Build history of the part. All positions in model axes, mm. A direction names the side the tool comes from. Coordinates: 2 decimals unless noted, no trailing zeros. Order: outer loops, then holes, each group sorted by start corner. A loop starts at its lowest first (then second) coordinate and runs counter-clockwise, first axis right, second up. Notation, with made-up numbers: M 13.25,70.25 L 33.25,70.25 A24 ccw 33.25,93.25 Z; hole C 22,-26.5 d6. An arc over 180 degrees is marked long. Write item = value, one per line. Start each with the question number.
Q1. Band-saw the part on A-A on x = 82. Write the cut outline in (y, z).
Q2. 3-axis set-ups, long thin cutter, end or side, ignore diameter. For faces 1 (the face through (-0.021, -62.935, 6.204)), 2 (the face through (80.5, -4.4, 3)), 3 (the face through (33, 0, 20)): which of +Z, -Z, +X, -X, +Y, -Y reach the whole face in a straight line?
Q3. Band-saw the part on D-D on x = 0. State how many separate pieces and enclosed holes the cut face has, plus the area to 3 significant figures.
Q4. Band-saw the part on C-C on z = 55.5. Write the cut outline in (x, y), plus the area to 3 significant figures.
Q5. Drill centre lines: probe 1 along Y at (x, z) = (0, 0.55); probe 2 along Y at (x, z) = (25.3, 55.5); probe 3 along Z at (x, y) = (25.55, 0). Where is each one in solid material? Low to high.
Q6. Pull direction X, two halves, no side cores. Call faces 4 (the face through (15, 16, 7)), 5 (the face through (0, -33, 20)), 6 (the face through (-25, 0, 10)): released by +X, released by -X, zero draft, split by the parting line, or undercut.
Q7. Pin check, flat tips, straight feed: P1, Ø11, axis at y = -39.5, z = 14.5, coming from the +X side; P2, Ø4, axis at y = 22.5, z = 17.5, coming from the +X side; P3, Ø2.5, axis at x = -3.5, z = 17.5, coming from the -Y side; P4, Ø3.5, axis at x = 23, y = 19, coming from the -Z side. Stop position of each tip, or through.
```python
from build123d import *

# Parameters (mm, degrees)
CROQUIS2_W                                           = 50
CROQUIS2_H                                           = 50
CROQUIS2_R                                           = 3.5
SALIENTE_EXTRUIR2_DEPTH                              = 20
CROQUIS3_R                                           = 7.5
CORTAR_EXTRUIR1_DEPTH                                = 3
SALIENTE_EXTRUIR3_DEPTH                              = 40
SALIENTE_EXTRUIR4_DEPTH                              = 2.65
CORTAR_EXTRUIR2_START                                = -2
CORTAR_EXTRUIR2_DEPTH                                = 5
CORTAR_EXTRUIR5_START                                = -2.65
CORTAR_EXTRUIR5_DEPTH                                = 2.65
SALIENTE_EXTRUIR5_DEPTH                              = 44.75
CROQUIS13_R                                          = 3
CORTAR_EXTRUIR6_DEPTH                                = 15.2
SALIENTE_EXTRUIR6_START                              = -21.5
SALIENTE_EXTRUIR6_DEPTH                              = 13
SALIENTE_EXTRUIR7_START                              = -5
SALIENTE_EXTRUIR7_DEPTH                              = 3
REDONDEO1_R                                          = 2
CROQUIS17_R                                          = 2
CORTAR_EXTRUIR7_DEPTH                                = 3
CROQUIS18_R                                          = 2
CORTAR_EXTRUIR8_DEPTH                                = 3
REFRENTADO_PARA_TORNILLO_TAP_N_CON_CABEZ_D           = 4.5
REFRENTADO_PARA_TORNILLO_TAP_N_CON_CABEZ_CSINK_D     = 8.96
REFRENTADO_PARA_TORNILLO_TAP_N_CON_CABEZ_CSINK_ANGLE = 90
REDONDEO1_OF_SIMETR_A3_R                             = 2


with BuildPart() as part:
    # Croquis2 → Saliente-Extruir2 (new body)
    with BuildSketch(Plane.XY):
        Rectangle(CROQUIS2_W, CROQUIS2_H)
        Circle(CROQUIS2_R, mode=Mode.SUBTRACT)
    extrude(amount=SALIENTE_EXTRUIR2_DEPTH)

    # Croquis3 → Cortar-Extruir1 (cut)
    with BuildSketch(Plane.XY.offset(20)):
        Circle(CROQUIS3_R)
    extrude(amount=-CORTAR_EXTRUIR1_DEPTH, mode=Mode.SUBTRACT)

    # Croquis4 → Saliente-Extruir3 (add)
    with BuildSketch(Plane(origin=(0, 0, 0), x_dir=(-1, 0, 0), z_dir=(0, 0, -1))):
        Polygon((-25, -25), (-25, 17.4), (-28, 17.4), (-28, -28), (17.4, -28), (17.4, -25), align=None)
    extrude(amount=-SALIENTE_EXTRUIR3_DEPTH)

    # Croquis5 → Saliente-Extruir4 (add)
    with BuildSketch(Plane(origin=(0, 17.4, 0), x_dir=(1, 0, 0), z_dir=(0, 1, 0))):
        Polygon((25, 0), (51, 0), (25, -25), align=None)
    saliente_extruir4 = extrude(amount=-SALIENTE_EXTRUIR4_DEPTH)

    # Croquis6 → Cortar-Extruir2 (cut)
    with BuildSketch(Plane.XZ.offset(-14.75).offset(CORTAR_EXTRUIR2_START)):
        Polygon((44.824955825, 4.550258722), (30.300169567, 18.516399355), (26.037550962, 14.083276006), (40.56233722, 0.117135373), align=None)
    cortar_extruir2 = extrude(amount=CORTAR_EXTRUIR2_DEPTH, mode=Mode.SUBTRACT)

    # Simetría2: Saliente-Extruir4, Cortar-Extruir2 across plane
    add(saliente_extruir4.mirror(Plane(origin=(0, 0, 0), x_dir=(0, 0, 1), z_dir=(0.707106781, 0.707106781, 0))))
    add(cortar_extruir2.mirror(Plane(origin=(0, 0, 0), x_dir=(0, 0, 1), z_dir=(0.707106781, 0.707106781, 0))), mode=Mode.SUBTRACT)

    # Croquis11 → Cortar-Extruir5 (cut)
    with BuildSketch(Plane.XZ.offset(-14.75).offset(CORTAR_EXTRUIR5_START)):
        Polygon((28, 0), (51, 0), (28, 22.115384615), align=None)
    extrude(amount=CORTAR_EXTRUIR5_DEPTH, mode=Mode.SUBTRACT)

    # Croquis14 → Saliente-Extruir5 (add)
    with BuildSketch(Plane.XZ.offset(-16.75)):
        Polygon((26.037550962, 14.083276006), (28, 12.196305777), (28, 16.124223005), align=None)
    extrude(amount=SALIENTE_EXTRUIR5_DEPTH)

    # Croquis13 → Cortar-Extruir6 (cut)
    with BuildSketch(Plane(origin=(0, 0, 0), x_dir=(-1, 0, 0), z_dir=(0, 0, -1))):
        with BuildLine():
            Line((-25, 25), (-14, 25))
            Line((-14, 25), (-14, 19))
            ThreePointArc((-14, 19), (-15.464466094, 15.464466094), (-19, 14))
            Line((-19, 14), (-25, 14))
            Line((-25, 14), (-28, 14))
            Line((-28, 14), (-28, 17.4))
            Line((-28, 17.4), (-25, 17.4))
            Line((-25, 17.4), (-25, 25))
        make_face()
        with Locations((-19.802765158, 19.802765158)):
            Circle(CROQUIS13_R, mode=Mode.SUBTRACT)
    extrude(amount=-CORTAR_EXTRUIR6_DEPTH, mode=Mode.SUBTRACT)

    # Croquis15 → Saliente-Extruir6 (add)
    with BuildSketch(Plane.XZ.offset(28).offset(SALIENTE_EXTRUIR6_START)):
        Polygon((28, 0), (78, 0), (89, 0), (89, 3), (75, 3), (28, 50), (28, 61), (25, 61), (25, 40), (28, 40), align=None)
        Polygon((31, 42.757359313), (70.757359313, 3), (31, 3), align=None, mode=Mode.SUBTRACT)
    saliente_extruir6 = extrude(amount=-SALIENTE_EXTRUIR6_DEPTH)

    # Croquis16 → Saliente-Extruir7 (add)
    with BuildSketch(Plane.XZ.offset(6.5).offset(SALIENTE_EXTRUIR7_START)):
        Polygon((31, 3), (70.757359313, 3), (31, 42.757359313), align=None)
        Polygon((33, 5), (65.928932188, 5), (33, 37.928932188), align=None, mode=Mode.SUBTRACT)
    saliente_extruir7 = extrude(amount=-SALIENTE_EXTRUIR7_DEPTH)

    # Redondeo1
    redondeo1_edges = [part.edges().sort_by_distance(p)[0] for p in [
        (33, 0, 37.928932188),
        (65.928932188, 0, 5),
        (33, 0, 5),
    ]]
    fillet(redondeo1_edges, radius=REDONDEO1_R)

    # Croquis17 → Cortar-Extruir7 (cut)
    with BuildSketch(Plane.XY.offset(3)):
        with Locations((82, 0)):
            Circle(CROQUIS17_R)
    cortar_extruir7 = extrude(amount=-CORTAR_EXTRUIR7_DEPTH, mode=Mode.SUBTRACT)

    # Croquis18 → Cortar-Extruir8 (cut)
    with BuildSketch(Plane(origin=(28, 0, 0), x_dir=(0, 0, -1), z_dir=(1, 0, 0))):
        with Locations((-55.5, 0)):
            Circle(CROQUIS18_R)
    cortar_extruir8 = extrude(amount=-CORTAR_EXTRUIR8_DEPTH, mode=Mode.SUBTRACT)

    # Refrentado para tornillo tap_n con cabez (through all)
    with Locations(Plane(origin=(28, 0, 0), x_dir=(0, 0, -1), z_dir=(1, 0, 0))):
        with Locations((-55.5, 0)):
            refrentado_para_tornillo_tap_n_con_cabez = CounterSinkHole(REFRENTADO_PARA_TORNILLO_TAP_N_CON_CABEZ_D / 2, REFRENTADO_PARA_TORNILLO_TAP_N_CON_CABEZ_CSINK_D / 2, counter_sink_angle=REFRENTADO_PARA_TORNILLO_TAP_N_CON_CABEZ_CSINK_ANGLE)

    # Croquis22 → Refrentado para tornillo tap_n con c 2 (revolve, cut)
    with BuildSketch(Plane(origin=(82, 0, 3), x_dir=(0, -1, 0), z_dir=(1, 0, 0))):
        Polygon((0, 0), (0, 3), (2.25, 3), (2.25, 2.23), (4.48, 0), align=None)
    refrentado_para_tornillo_tap_n_con_c_2 = revolve(axis=Axis((82, 0, 9.35), (0, 0, -1)), mode=Mode.SUBTRACT)

    # Simetría3: Saliente-Extruir6, Saliente-Extruir7, Cortar-Extruir7, Cortar-Extruir8, Refrentado para tornillo tap_n con cabez, Refrentado para tornillo tap_n con c 2 across plane
    add(saliente_extruir6.mirror(Plane(origin=(0, 0, 0), x_dir=(0, 0, 1), z_dir=(0.707106781, 0.707106781, 0))))
    add(saliente_extruir7.mirror(Plane(origin=(0, 0, 0), x_dir=(0, 0, 1), z_dir=(0.707106781, 0.707106781, 0))))
    add(cortar_extruir7.mirror(Plane(origin=(0, 0, 0), x_dir=(0, 0, 1), z_dir=(0.707106781, 0.707106781, 0))), mode=Mode.SUBTRACT)
    add(cortar_extruir8.mirror(Plane(origin=(0, 0, 0), x_dir=(0, 0, 1), z_dir=(0.707106781, 0.707106781, 0))), mode=Mode.SUBTRACT)
    add(refrentado_para_tornillo_tap_n_con_cabez.mirror(Plane(origin=(0, 0, 0), x_dir=(0, 0, 1), z_dir=(0.707106781, 0.707106781, 0))), mode=Mode.SUBTRACT)
    add(refrentado_para_tornillo_tap_n_con_c_2.mirror(Plane(origin=(0, 0, 0), x_dir=(0, 0, 1), z_dir=(0.707106781, 0.707106781, 0))), mode=Mode.SUBTRACT)

    # Redondeo1 of Simetría3
    redondeo1_of_simetr_a3_edges = [part.edges().sort_by_distance(p)[0] for p in [
        (0, -33, 37.928932188),
        (0, -65.928932188, 5),
        (0, -33, 5),
    ]]
    fillet(redondeo1_of_simetr_a3_edges, radius=REDONDEO1_OF_SIMETR_A3_R)


solid = part.part
```
Recorded:
q1.outline = M -6.5,0 L -2.25,0 L -2.25,0.77 L -4.48,3 L -6.5,3 Z; M 2.25,0 L 6.5,0 L 6.5,3 L 4.48,3 L 2.25,0.77 Z
q2.face_1 = +X, -X
q2.face_2 = +Z, +X, +Y, -Y
q2.face_3 = +Y, -Y
q3.separate_pieces = 4
q3.enclosed_holes = 1
q3.area = 1,740 mm2
q4.outline = M -6.5,-28 L -4.48,-28 L -2.25,-25.77 L -2.25,-25 L -6.5,-25 Z; M 2.25,-25.77 L 4.48,-28 L 6.5,-28 L 6.5,-25 L 2.25,-25 Z; M 25,-6.5 L 28,-6.5 L 28,-4.48 L 25.77,-2.25 L 25,-2.25 Z; M 25,2.25 L 25.77,2.25 L 28,4.48 L 28,6.5 L 25,6.5 Z
q4.area = 41.1 mm2
q5.probe_1 = -89 to -84.25, -79.75 to -3.5, 3.5 to 25
q5.probe_2 = -6.5 to -2.25, 2.25 to 6.5
q5.probe_3 = 0 to 53.25, 57.75 to 61
q6.face_4 = undercut
q6.face_5 = zero draft
q6.face_6 = released by -X
q7.P1 = -14.75
q7.P2 = 25
q7.P3 = -61.75
q7.P4 = 0
